Design review of the part built by this model. Coordinates are the model's own, in mm. A direction names the side the tool comes from. Give positions to 0.01 mm unless a question says otherwise; leave off trailing zeros. Write each loop counter-clockwise with the first axis right and the second up, starting at its lowest first coordinate (ties: lowest second). Pieces come first, ordered by that corner, then holes. Notation, with made-up numbers: (50, 32.5) -> (95, 32.5) arc R24 ccw to (95, 60.5) -> close; hole circle Ø7 at (-16.5, 40). An arc over 180 degrees is marked (long way). Answer as a JSON object with one key per item and string values.
```python
from build123d import *

# Parameters (mm, degrees)
SKETCH1_W           = 20
SKETCH1_H           = 30
BOSS_EXTRUDE1_DEPTH = 30
SKETCH2_W           = 10
SKETCH2_H           = 20
CUT_EXTRUDE1_DEPTH  = 25
SKETCH3_W           = 30
SKETCH3_H           = 8
BOSS_EXTRUDE2_DEPTH = 3
LPATTERN1_COUNT     = 8
LPATTERN1_PITCH     = 23
SKETCH4_W           = 30
SKETCH4_H           = 22
BOSS_EXTRUDE3_DEPTH = 3
SKETCH5_W           = 30
SKETCH5_H           = 30
BOSS_EXTRUDE4_DEPTH = 3
SKETCH6_W           = 151
SKETCH6_H           = 3
CUT_EXTRUDE2_DEPTH  = 3
SKETCH7_W           = 187
SKETCH7_H           = 30
BOSS_EXTRUDE5_DEPTH = 5


with BuildPart() as part:
    # Sketch1 → Boss-Extrude1 (new body)
    with BuildSketch(Plane.XY):
        with Locations((10, 15)):
            Rectangle(SKETCH1_W, SKETCH1_H)
    extrude(amount=BOSS_EXTRUDE1_DEPTH)

    # Sketch2 → Cut-Extrude1 (cut)
    with BuildSketch(Plane.XZ):
        with Locations((10, 15)):
            Rectangle(SKETCH2_W, SKETCH2_H)
    extrude(amount=-CUT_EXTRUDE1_DEPTH, mode=Mode.SUBTRACT)

    # Sketch3 → Boss-Extrude2 (add)
    with BuildSketch(Plane(origin=(20, 0, 0), x_dir=(0, 0, -1), z_dir=(1, 0, 0))):
        with Locations((-15, 4)):
            Rectangle(SKETCH3_W, SKETCH3_H)
    extrude(amount=BOSS_EXTRUDE2_DEPTH)


with BuildPart() as lpattern1_1:
    # LPattern1: pattern copy
    add(part.part.moved(Location(Vector(1, 0, 0) * (1 * LPATTERN1_PITCH))))


with BuildPart() as lpattern1_2:
    # LPattern1: pattern copy
    add(part.part.moved(Location(Vector(1, 0, 0) * (2 * LPATTERN1_PITCH))))


with BuildPart() as lpattern1_3:
    # LPattern1: pattern copy
    add(part.part.moved(Location(Vector(1, 0, 0) * (3 * LPATTERN1_PITCH))))


with BuildPart() as lpattern1_4:
    # LPattern1: pattern copy
    add(part.part.moved(Location(Vector(1, 0, 0) * (4 * LPATTERN1_PITCH))))


with BuildPart() as lpattern1_5:
    # LPattern1: pattern copy
    add(part.part.moved(Location(Vector(1, 0, 0) * (5 * LPATTERN1_PITCH))))


with BuildPart() as lpattern1_6:
    # LPattern1: pattern copy
    add(part.part.moved(Location(Vector(1, 0, 0) * (6 * LPATTERN1_PITCH))))


with BuildPart() as lpattern1_7:
    # LPattern1: pattern copy
    add(part.part.moved(Location(Vector(1, 0, 0) * (7 * LPATTERN1_PITCH))))

    # Combine1: union part, LPattern1_1, LPattern1_2, LPattern1_3, LPattern1_4, LPattern1_5, LPattern1_6
    add(part.part)
    add(lpattern1_1.part)
    add(lpattern1_2.part)
    add(lpattern1_3.part)
    add(lpattern1_4.part)
    add(lpattern1_5.part)
    add(lpattern1_6.part)

    # Sketch4 → Boss-Extrude3 (add)
    with BuildSketch(Plane(origin=(181, 0, 0), x_dir=(0, 0, -1), z_dir=(1, 0, 0))):
        with Locations((-15, 19)):
            Rectangle(SKETCH4_W, SKETCH4_H)
    extrude(amount=BOSS_EXTRUDE3_DEPTH)

    # Sketch5 → Boss-Extrude4 (add)
    with BuildSketch(Plane.ZY):
        with Locations((15, 15)):
            Rectangle(SKETCH5_W, SKETCH5_H)
    extrude(amount=BOSS_EXTRUDE4_DEPTH)

    # Sketch6 → Cut-Extrude2 (cut)
    with BuildSketch(Plane.XZ):
        with Locations((90.5, 15)):
            Rectangle(SKETCH6_W, SKETCH6_H)
    extrude(amount=-CUT_EXTRUDE2_DEPTH, mode=Mode.SUBTRACT)

    # Sketch7 → Boss-Extrude5 (add)
    with BuildSketch(Plane.XZ):
        with Locations((90.5, 15)):
            Rectangle(SKETCH7_W, SKETCH7_H)
    extrude(amount=BOSS_EXTRUDE5_DEPTH)


solid = lpattern1_7.part
```
(1) For line 1 along Z through (x, y) = (97.5, 7); line 2 along Y through (x, z) = (57.5, 19); line 3 along Y through (x, z) = (160, 3), list the stretches that pass through material, from the lowest coordinate up.
Here are the results:
{"line 1": "z = 0 to 5, 25 to 30", "line 2": "y = -5 to 0, 25 to 30", "line 3": "y = -5 to 8"}
(2) We need section A-A, the plane x = 77.5. State the section outline as (y, z) points, then the cut area to 3 significant figures.
Here are the results:
{"outline": "(-5, 0) -> (30, 0) -> (30, 30) -> (-5, 30) -> close; hole (0, 5) -> (25, 5) -> (25, 25) -> (0, 25) -> close", "area": "550 mm²"}
(3) For faces 5 (the flat face through (9, 30, 15)), 6 (the flat face through (44, 1, 16.5)), 7 (the flat face through (159, 8, 15)), list the 3-axis set-ups (+Z, -Z, +X, -X, +Y, -Y) from which the entire face can be reached by the end or side of a thin tool; tool diameter is ignored.
Here are the results:
{"face 5": "+Z, -Z, +X, -X, +Y", "face 6": "none", "face 7": "+Z, -Z, +Y"}
(4) The part is to be moulded in two halves that separate along Z. For faces 1 (the flat face through (130, 12, 15)), 2 (the flat face through (159, 1, 13.5)), 3 (the flat face through (23, 19, 15)), 4 (the flat face through (89, 5, 30)), say which applies: +Z half, -Z half, draft (parallel to the pull), parting line (faces both ways), or undercut.
Here are the results:
{"face 1": "undercut", "face 2": "undercut", "face 3": "draft", "face 4": "+Z half"}
(5) Clearance check with a flat-ended pin moving along its axis: pin 1 (2.5 mm diameter, centred on x = 44.5, z = 17.5, fed in from +Y). State where the tip first meets the part, or that it passes through.
Here are the results:
{"pin 1": "stops at y = 8"}
(6) We need section B-B, the plane y = 22.5. Give the number of separate pieces and of enclosed holes in the cut face, then the cut area to 3 significant figures.
Here are the results:
{"separate pieces": "8", "enclosed holes": "8", "area": "3,380 mm²"}
